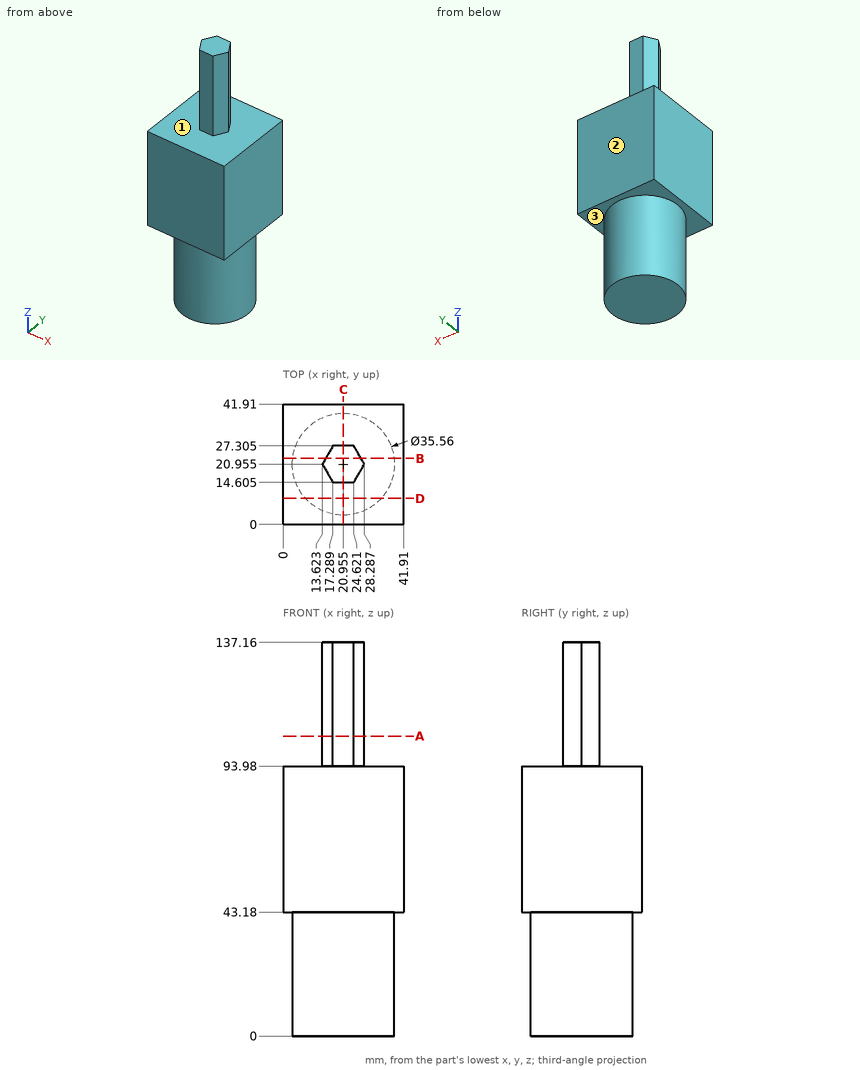
Could you check a few things on this drawing? It's one solid part, dimensions in mm from its lowest x, y, z. A direction names the side the tool comes from. Give positions to 0.01 mm unless a question says otherwise; leave off trailing zeros. Order: outer loops, then holes, each group sorted by start corner. A loop starts at its lowest first (then second) coordinate and runs counter-clockwise, first axis right, second up.
1. Suppose I cut it at A-A (z = 104.5). Write out the boundary of the cut face in (x, y) (1 decimal).
Answers below:
outline: (13.6, 21) - (17.3, 14.6) - (24.6, 14.6) - (28.3, 21) - (24.6, 27.3) - (17.3, 27.3) - close
2. Which directions (+Z, -Z, +X, -X, +Y, -Y) give clear straight access to the entire face, cutting with the end or side of a thin tool? Please do the marked faces 1, 2 and 3.
Answers below:
face 1: +Z
face 2: +Z, -Z, +X, -X, +Y
face 3: -Z
3. I need wall thicknesses on L1, parallel to Z at x = 14, y = 25; L2, parallel to Z at x = 40, y = 24; L3, parallel to X at y = 4.5, z = 21. Which ranges of each line are inside material? Lowest first, please.
Answers below:
L1: z = 0 to 93.98
L2: z = 43.18 to 93.98
L3: x = 14.22 to 27.69
4. Suppose I cut it at B-B (y = 23). Write out the boundary of the cut face in (x, z), plus the area to 3 significant figures.
Answers below:
outline: (0, 43.18) - (3.29, 43.18) - (3.29, 0) - (38.62, 0) - (38.62, 43.18) - (41.91, 43.18) - (41.91, 93.98) - (27.11, 93.98) - (27.11, 137.16) - (14.8, 137.16) - (14.8, 93.98) - (0, 93.98) - close
area: 4,190 mm2
5. For pin 1 (8 mm diameter, centred on x = 21, z = 115, fed in from +Y) (3 decimals); pin 2 (6 mm diameter, centred on x = 22.5, z = 107, fed in from -Y) (3 decimals); pin 3 (3 mm diameter, centred on x = 26, y = 11, fed in from +Z), each with a flat end and sliding along its axis, tell me the tip position at first contact or that it passes through.
Answers below:
pin 1: stops at y = 27.305
pin 2: stops at y = 14.605
pin 3: stops at z = 93.98
6. Suppose I cut it at C-C (x = 21). Write out the boundary of the cut face in (y, z) (1 decimal).
Answers below:
outline: (0, 43.2) - (3.2, 43.2) - (3.2, 0) - (38.7, 0) - (38.7, 43.2) - (41.9, 43.2) - (41.9, 94) - (27.3, 94) - (27.3, 137.2) - (14.6, 137.2) - (14.6, 94) - (0, 94) - close
7. Suppose I cut it at D-D (y = 9). Write out the boundary of the cut face in (x, z).
Answers below:
outline: (0, 43.18) - (7.79, 43.18) - (7.79, 0) - (34.12, 0) - (34.12, 43.18) - (41.91, 43.18) - (41.91, 93.98) - (0, 93.98) - close
